Build history of the part. All positions in model axes, mm. A direction names the side the tool comes from. Coordinates: 2 decimals unless noted, no trailing zeros. Loops run counter-clockwise (first coordinate to the right, second up) from the corner with the lowest first, then second, coordinate; pieces in that order, holes last.
Item 1: 3-axis set-ups, long thin cutter, end or side, ignore diameter. For faces 1 (the face through (9, 1, -4)), 2 (the face through (0, 1, -6)), 3 (the face through (3.26, 4.014, -4.776)): which of +Z, -Z, +X, -X, +Y, -Y reach the whole face in a straight line?
Item 2: Flat gauge pins, fed straight in: pin 1 (3 mm diameter, centred on y = 2, z = -9.5, fed in from +X); pin 2 (1.2 mm diameter, centred on y = 3, z = -6.5, fed in from +X). Where does each tip first touch, or does it go through?
Item 3: Cut at A-A (x = 8). List the corners of the cut face in (y, z), and give its area (3 significant figures).
Item 4: Cut at C-C (y = 1.7). List the corners of the cut face in (x, z).
Item 5: Cut at D-D (z = -6.5). List the corners of the cut face in (x, y).
Item 6: Mould opens along Z. For faces 4 (the face through (3, 1, -6)), 5 (the face through (12, 3, -2)), 6 (the face through (6, 3, 0)), 7 (the face through (3.26, 2.01, -4.76)) say: released by +Z, released by -Z, zero draft, split by the parting line, or undercut.
Item 7: Cut at B-B (z = -1.5). List the corners of the cut face in (x, y), and give its area (3 significant figures).
Item 8: Drill centre lines: line 1 along Y through (x, z) = (8, -1.6); line 2 along Y through (x, z) = (1.9, -6.5); line 3 along X through (y, z) = (2.6, -8.75). Where is each one in solid material? Low to high.
from build123d import *

# Parameters (mm, degrees)
EXTRUDE_1_DEPTH     = 5.5
CUT_EXTRUDE_1_REACH = 19.84
SKETCH_2_R          = 1
CUT_EXTRUDE_2_DEPTH = 1.5
CUT_EXTRUDE_3_REACH = 17.435
SKETCH_4_R          = 1.35


with BuildPart() as part:
    # 草图1 → 凸台-拉伸1 (new body)
    with BuildSketch(Plane(origin=(0, 0, 0), x_dir=(1, 0, 0), z_dir=(0, 1, 0))):
        Polygon((0, 0), (12, 0), (12, 4), (4, 4), (4, 12), (0, 12), align=None)
    extrude(amount=EXTRUDE_1_DEPTH)

    # 草图2 → 切除-拉伸1 (cut, up to next)
    with BuildSketch(Plane.ZY, mode=Mode.PRIVATE) as cut_extrude_1_sk1:
        with Locations((-6.5, 3)):
            Circle(SKETCH_2_R)
    cut_extrude_1_tool1 = extrude(cut_extrude_1_sk1.sketch, amount=-CUT_EXTRUDE_1_REACH, mode=Mode.PRIVATE) & part.part
    add(cut_extrude_1_tool1.solids().sort_by_distance((0, 3, -6.5))[0], mode=Mode.SUBTRACT)

    # 草图3 → 切除-拉伸2 (cut)
    with BuildSketch(Plane(origin=(4, 0, 0), x_dir=(0, 0, -1), z_dir=(1, 0, 0))):
        Polygon((8.809401077, 3), (7.654700538, 5), (5.345299462, 5), (4.190598923, 3), (5.345299462, 1), (7.654700538, 1), align=None)
    extrude(amount=-CUT_EXTRUDE_2_DEPTH, mode=Mode.SUBTRACT)

    # 草图4 → 切除-拉伸3 (cut, up to next)
    with BuildSketch(Plane(origin=(0, 0, -4), x_dir=(-1, 0, 0), z_dir=(0, 0, -1)), mode=Mode.PRIVATE) as cut_extrude_3_sk1:
        with Locations((-8, 2.75)):
            Circle(SKETCH_4_R)
    cut_extrude_3_tool1 = extrude(cut_extrude_3_sk1.sketch, amount=-CUT_EXTRUDE_3_REACH, mode=Mode.PRIVATE) & part.part
    add(cut_extrude_3_tool1.solids().sort_by_distance((8, 2.75, -4))[0], mode=Mode.SUBTRACT)


solid = part.part
Filled sheet:
1. face 1: -Z, +X, +Y, -Y
1. face 2: +Z, -Z, -X, +Y, -Y
1. face 3: +X
2. pin 1: stops at x = 4
2. pin 2: passes through
3. outline: (0, -4) - (1.4, -4) - (1.4, 0) - (0, 0) - close; (4.1, -4) - (5.5, -4) - (5.5, 0) - (4.1, 0) - close
3. area: 11.2 mm2
4. outline: (0, -12) - (4, -12) - (4, -8.06) - (2.5, -8.06) - (2.5, -4.94) - (4, -4.94) - (4, -4) - (7.15, -4) - (7.15, 0) - (0, 0) - close; (8.85, -4) - (12, -4) - (12, 0) - (8.85, 0) - close
5. outline: (0, 0) - (4, 0) - (4, 1) - (2.5, 1) - (2.5, 2) - (0, 2) - close; (0, 4) - (2.5, 4) - (2.5, 5) - (4, 5) - (4, 5.5) - (0, 5.5) - close
6. face 4: undercut
6. face 5: zero draft
6. face 6: released by +Z
6. face 7: undercut
7. outline: (0, 0) - (12, 0) - (12, 5.5) - (0, 5.5) - close; hole circle Ø2.7 at (8, 2.75)
7. area: 60.3 mm2
8. line 1: y = 0 to 1.4, 4.1 to 5.5
8. line 2: y = 0 to 2, 4 to 5.5
8. line 3: x = 0 to 4
